from build123d import *

# Parameters (mm, degrees)
SKETCH3_R                       = 4.7625
BOSS_EXTRUDE1_DEPTH             = 150
BOSS_EXTRUDE1_DIRECTION_2_REACH = 54.926
BOSS_EXTRUDE2_DEPTH             = 1.5875
SKETCH5_R                       = 3.175
CUT_EXTRUDE1_DEPTH              = 183.813192428


with BuildPart() as part:
    # Sketch1 → Revolve1 (revolve)
    with BuildSketch(Plane.XY, mode=Mode.PRIVATE) as revolve1_sk:
        Polygon((-28.575, 12.7), (9.525, 12.7), (9.525, 6.35), (3.175, 6.35), (3.175, 3.01625), (-15.875, 3.01625), (-15.875, 6.35), (-28.575, 6.35), align=None)
    revolve(revolve1_sk.sketch.rotate(Axis((-58.643350072, 0, 0), (1, 0, 0)), 90), axis=Axis((-58.643350072, 0, 0), (1, 0, 0)))

    # Sketch3 → Boss-Extrude1 (add)
    with BuildSketch(Plane(origin=(0, 30, 0), x_dir=(-1, 0, 0), z_dir=(0, 1, 0))):
        with Locations(Location((0, 0, 0), (0, 0, 90))):
            Circle(SKETCH3_R)
    extrude(amount=BOSS_EXTRUDE1_DEPTH)

    # Sketch3 → Boss-Extrude1 direction 2 (add, up to next)
    with BuildSketch(Plane(origin=(0, 30, 0), x_dir=(-1, 0, 0), z_dir=(0, 1, 0)), mode=Mode.PRIVATE) as boss_extrude1_direction_2_sk1:
        with Locations(Location((0, 0, 0), (0, 0, 90))):
            Circle(SKETCH3_R)
    boss_extrude1_direction_2_tool1 = extrude(boss_extrude1_direction_2_sk1.sketch, amount=-BOSS_EXTRUDE1_DIRECTION_2_REACH, mode=Mode.PRIVATE) - part.part
    add(boss_extrude1_direction_2_tool1.solids().sort_by_distance((0, 30, 0))[0])

    # Sketch4 → Boss-Extrude2 (add, symmetric)
    with BuildSketch(Plane.XY):
        with BuildLine():
            Line((-3.175, 11.1125), (-22.225, 11.1125))
            Line((-22.225, 11.1125), (-22.225, 23.8125))
            ThreePointArc((-22.225, 23.8125), (-20.365128061, 28.302628061), (-15.875, 30.1625))
            Line((-15.875, 30.1625), (-3.175, 30.1625))
            Line((-3.175, 30.1625), (-3.175, 11.1125))
        make_face()
    extrude(amount=BOSS_EXTRUDE2_DEPTH, both=True)

    # Sketch5 → Cut-Extrude1 (cut, through all)
    with BuildSketch(Plane.XY.offset(1.5875)):
        with Locations((-15.875, 23.8125)):
            Circle(SKETCH5_R)
    extrude(amount=-CUT_EXTRUDE1_DEPTH, mode=Mode.SUBTRACT)


solid = part.part
Input: part model. Units: mm. Frame: model coordinates. A direction names the side the tool comes from. Coordinates: 2 decimals unless noted, no trailing zeros. Loops run counter-clockwise (first coordinate to the right, second up) from the corner with the lowest first, then second, coordinate; pieces in that order, holes last. Notation, with made-up numbers: (42.5, -24.5) -> (72.5, -24.5) arc R19 cw to (72.5, 10.5) -> close; hole circle Ø6 at (38, 43.5). An arc over 180 degrees is marked (long way). One line per item, written item: value.
(1) Draft query along Z for faces 5 (the face through (-22.225, 18, 0)), 6 (the face through (3.175, -2, 3)), 7 (the face through (4.016, 97.064, 2.56)). Return one class per face: pulls with the +Z half, pulls with the -Z half, needs draft (parallel to the pull), parting line crosses it, or undercut.
Answer below:
face 5: needs draft
face 6: undercut
face 7: parting line crosses it
(2) Cut plane B-B (y = 0). Output: boundary loops of the cut face in (x, z) (3 decimals), then the cut area to 3 significant figures.
Answer below:
outline: (-28.575, -12.7) -> (9.525, -12.7) -> (9.525, -6.35) -> (3.175, -6.35) -> (3.175, -3.016) -> (-15.875, -3.016) -> (-15.875, -6.35) -> (-28.575, -6.35) -> close; (-28.575, 6.35) -> (-15.875, 6.35) -> (-15.875, 3.016) -> (3.175, 3.016) -> (3.175, 6.35) -> (9.525, 6.35) -> (9.525, 12.7) -> (-28.575, 12.7) -> close
area: 611 mm2
(3) Cut plane D-D (y = 77.5). Output: boundary loops of the cut face in (x, z) (1 decimal), then the cut area to 3 significant figures.
Answer below:
outline: circle Ø9.5 at (0, 0)
area: 71.3 mm2
(4) Cut plane C-C (x = -10). Output: boundary loops of the cut face in (y, z), then the cut area to 3 significant figures.
Answer below:
outline: (12.6, -1.59) -> (30.16, -1.59) -> (30.16, 1.59) -> (12.6, 1.59) arc R12.7 ccw (long way) to start; hole circle Ø6.03 at (0, 0)
area: 534 mm2
(5) Cut plane A-A (z = 0). Give the number of separate pieces and of enclosed holes in the cut face, then the cut area to 3 significant figures.
Answer below:
separate pieces: 2
enclosed holes: 1
area: 2,470 mm2
(6) Set-up query: faces 1 (the face through (-13, 22, -1.588)), 2 (the face through (-13, 22, 1.588)), 3 (the face through (6.31, 3.86, -5.04)), 4 (the face through (-15.875, -2, -3)). Return all of +Z, -Z, +X, -X, +Y, -Y with unobstructed straight access to the full face (end or side cutting, diameter ignored); none if empty.
Answer below:
face 1: -Z, -X, +Y
face 2: +Z, -X, +Y
face 3: +X
face 4: -X
(7) Pin query (flat end, axial travel): pin 1 Ø6.5 at (y, z) = (1.5, 1.5) entering from +X (3 decimals); pin 2 Ø8.5 at (x, y) = (-15.88, 23.81) entering from +Z; pin 3 Ø1.5 at (x, z) = (-13, -3.5) entering from -Y. Return the tip coordinate at first contact, or that it passes through.
Answer below:
pin 1: stops at x = 3.175
pin 2: stops at z = 1.59
pin 3: stops at y = -12.4
(8) Ray query, line 1 along Y through (x, z) = (-10.5, 0); line 2 along Y through (x, z) = (6.5, 0); line 3 along Z through (x, y) = (-11, 15.5). Return the intervals inside material, ascending.
Answer below:
line 1: y = -12.7 to -3.02, 3.02 to 30.16
line 2: y = -12.7 to -6.35, 6.35 to 12.7
line 3: z = -1.59 to 1.59
